```python
from build123d import *

# Parameters (mm, degrees)
AUFSATZ_LINEAR_AUSTRAGEN1_DEPTH      = 2.5
AUFSATZ_LINEAR_AUSTRAGEN1_DEPTH_BACK = 2.5
SKIZZE2_R                            = 1.5
SCHNITT_LINEAR_AUSTRAGEN1_DEPTH      = 3.5
SCHNITT_LINEAR_AUSTRAGEN1_DEPTH_BACK = 3.5
SCHNITT_LINEAR_AUSTRAGEN2_DEPTH      = 3.5
SCHNITT_LINEAR_AUSTRAGEN2_DEPTH_BACK = 3.5
SKIZZE7_W                            = 50
SKIZZE7_H                            = 20
AUFSATZ_LINEAR_AUSTRAGEN3_DEPTH      = 10
SCHNITT_LINEAR_AUSTRAGEN6_DEPTH      = 13.5
FASE1_SIZE                           = 2
SKETCH1_R                            = 3.175
CUT_EXTRUDE1_DEPTH                   = 10
SKETCH2_W                            = 15
SKETCH2_H                            = 3.5
BOSS_EXTRUDE1_DEPTH                  = 2.225
FILLET2_R                            = 5
FILLET1_R                            = 2


with BuildPart() as part:
    # Skizze1 → Aufsatz-Linear austragen1 (new body, two sides)
    with BuildSketch(Plane.XY) as aufsatz_linear_austragen1_sk:
        Polygon((-50, -20), (-50, 20), (50, 20), (50, -20), (25, -20), (25, -40), (-25, -40), (-25, -20), align=None)
    extrude(amount=AUFSATZ_LINEAR_AUSTRAGEN1_DEPTH)
    extrude(aufsatz_linear_austragen1_sk.sketch, amount=-AUFSATZ_LINEAR_AUSTRAGEN1_DEPTH_BACK)

    # Skizze2 → Schnitt-Linear austragen1 (cut, two sides)
    with BuildSketch(Plane.XY) as schnitt_linear_austragen1_sk:
        with Locations((-45, 15)):
            Circle(SKIZZE2_R)
        with Locations((-45, -15)):
            Circle(SKIZZE2_R)
        with Locations((45, -15)):
            Circle(SKIZZE2_R)
        with Locations((45, 15)):
            Circle(SKIZZE2_R)
    extrude(amount=SCHNITT_LINEAR_AUSTRAGEN1_DEPTH, mode=Mode.SUBTRACT)
    extrude(schnitt_linear_austragen1_sk.sketch, amount=-SCHNITT_LINEAR_AUSTRAGEN1_DEPTH_BACK, mode=Mode.SUBTRACT)

    # Skizze4 → Schnitt-Linear austragen2 (cut, two sides)
    with BuildSketch(Plane.XY) as schnitt_linear_austragen2_sk:
        with BuildLine():
            Line((-48, -8), (-48, 8))
            ThreePointArc((-48, 8), (-47.121320344, 10.121320344), (-45, 11))
            Line((-45, 11), (-40.5, 11))
            ThreePointArc((-40.5, 11), (-38.378679656, 10.121320344), (-37.5, 8))
            Line((-37.5, 8), (-37.5, -8))
            ThreePointArc((-37.5, -8), (-38.378679656, -10.121320344), (-40.5, -11))
            Line((-40.5, -11), (-45, -11))
            ThreePointArc((-45, -11), (-47.121320344, -10.121320344), (-48, -8))
        make_face()
        with BuildLine():
            Line((45, -11), (40.5, -11))
            ThreePointArc((40.5, -11), (38.378679656, -10.121320344), (37.5, -8))
            Line((37.5, -8), (37.5, 8))
            ThreePointArc((37.5, 8), (38.378679656, 10.121320344), (40.5, 11))
            Line((40.5, 11), (45, 11))
            ThreePointArc((45, 11), (47.121320344, 10.121320344), (48, 8))
            Line((48, 8), (48, -8))
            ThreePointArc((48, -8), (47.121320344, -10.121320344), (45, -11))
        make_face()
    extrude(amount=SCHNITT_LINEAR_AUSTRAGEN2_DEPTH, mode=Mode.SUBTRACT)
    extrude(schnitt_linear_austragen2_sk.sketch, amount=-SCHNITT_LINEAR_AUSTRAGEN2_DEPTH_BACK, mode=Mode.SUBTRACT)

    # Skizze7 → Aufsatz-Linear austragen3 (add)
    with BuildSketch(Plane(origin=(0, 0, -2.5), x_dir=(-1, 0, 0), z_dir=(0, 0, -1))):
        with Locations((0, -30)):
            Rectangle(SKIZZE7_W, SKIZZE7_H)
        Polygon((35, 20), (-35, 20), (-35, -20), (-25, -20), (25, -20), (35, -20), align=None)
    extrude(amount=AUFSATZ_LINEAR_AUSTRAGEN3_DEPTH)

    # Skizze8 → Schnitt-Linear austragen6 (cut)
    with BuildSketch(Plane.XY.offset(2.5)):
        with BuildLine():
            Line((30, 18), (-30, 18))
            ThreePointArc((-30, 18), (-32.121320344, 17.121320344), (-33, 15))
            Line((-33, 15), (-33, -15))
            ThreePointArc((-33, -15), (-32.121320344, -17.121320344), (-30, -18))
            Line((-30, -18), (30, -18))
            ThreePointArc((30, -18), (32.121320344, -17.121320344), (33, -15))
            Line((33, -15), (33, 15))
            ThreePointArc((33, 15), (32.121320344, 17.121320344), (30, 18))
        make_face()
        with BuildLine():
            Line((23, -18), (-23, -18))
            Line((-23, -18), (-23, -35))
            ThreePointArc((-23, -35), (-22.121320344, -37.121320344), (-20, -38))
            Line((-20, -38), (20, -38))
            ThreePointArc((20, -38), (22.121320344, -37.121320344), (23, -35))
            Line((23, -35), (23, -18))
        make_face()
    extrude(amount=-SCHNITT_LINEAR_AUSTRAGEN6_DEPTH, mode=Mode.SUBTRACT)

    # Fase1
    fase1_edges = [part.edges().sort_by_distance(p)[0] for p in [
        (-50, -20, 0),
        (-50, 20, 0),
        (50, 20, 0),
        (50, -20, 0),
        (25, -40, -5),
        (-25, -40, -5),
    ]]
    chamfer(fase1_edges, length=FASE1_SIZE)

    # Sketch1 → Cut-Extrude1 (cut)
    with BuildSketch(Plane(origin=(0, -40, 0), x_dir=(1, 0, 0), z_dir=(0, 1, 0))):
        with Locations((0, 4.25)):
            Circle(SKETCH1_R)
    extrude(amount=CUT_EXTRUDE1_DEPTH, mode=Mode.SUBTRACT)

    # Sketch2 → Boss-Extrude1 (add)
    with BuildSketch(Plane.XY.offset(-11)):
        with Locations((0, -36.25)):
            Rectangle(SKETCH2_W, SKETCH2_H)
    extrude(amount=BOSS_EXTRUDE1_DEPTH)

    # Fillet2
    fillet2_edges = [part.edges().sort_by_distance(p)[0] for p in [
        (-35, 0, -12.5),
        (35, 0, -12.5),
    ]]
    fillet(fillet2_edges, radius=FILLET2_R)

    # Fillet1
    fillet1_edges = [part.edges().sort_by_distance(p)[0] for p in [
        (-7.5, -36.25, -11),
        (7.5, -36.25, -11),
        (0, -34.5, -11),
    ]]
    fillet(fillet1_edges, radius=FILLET1_R)


solid = part.part
```
Geometry check sheet. Reference: the model listing, model coordinates, mm. A direction names the side the tool comes from. Coordinates: 2 decimals unless noted, no trailing zeros. Order: outer loops, then holes, each group sorted by start corner. A loop starts at its lowest first (then second) coordinate and runs counter-clockwise, first axis right, second up.
Item 1: Section check C-C (x = -19). Enter the section's corners in (y, z).
Item 2: Mould release check, pull along Z, two halves, no side actions. Record for faces 5 (the cylindrical face through (-8.1, -35.82, -10.43)), 6 (the cylindrical face through (-0.69, -39.01, -1.15)), 7 (the flat face through (35, 0, -5)): released by +Z, released by -Z, zero draft, split by the parting line, or undercut.
Item 3: Section check A-A (x = 0). Enter the section's corners in (y, z) (3 decimals).
Item 4: Scan lines: line 1 along Y through (x, z) = (-45, -1.05); line 2 along X through (y, z) = (15, 0.55); line 3 along X through (y, z) = (-26, -10.25). Record each from-to range of solid material in increasing order.
Item 5: Section check D-D (y = 9). Enter the section's corners in (x, z).
Item 6: Tool access check on faces 1 (the flat face through (-34, -20, -3)), 2 (the flat face through (24, -39, -5)), 3 (the cylindrical face through (-47.14, 10.1, 0.04)), 4 (the cylindrical face through (22.1, -37.14, -4.16)). Record the directions out of +Z, -Z, +X, -X, +Y, -Y that give a thin tool (end or side, any length) a straight path to the whole face; none if there is none.
Item 7: Depth check by flat-ended pin: pin 1 (1.3 mm diameter, centred on x = -42.5, z = 0.5, fed in from -Y); pin 2 (2.5 mm diameter, centred on x = -45, y = 15, fed in from -Z); pin 3 (6 mm diameter, centred on y = -26, z = -2.5, fed in from -X); pin 4 (7.5 mm diameter, centred on y = -33, z = -3, fed in from +X). Enter the tip coordinate at first touch or a pass-through.
Item 8: Section check B-B (y = 3). Enter the section's corners in (x, z).
Check sheet entries:
1. outline: (-40, -12.5) - (20, -12.5) - (20, 2.5) - (18, 2.5) - (18, -11) - (-38, -11) - (-38, 2.5) - (-40, 2.5) - close
2. face 5: released by +Z
2. face 6: undercut
2. face 7: zero draft
3. outline: (-40, -12.5) - (20, -12.5) - (20, 2.5) - (18, 2.5) - (18, -11) - (-32.5, -11) arc R2 cw to (-34.5, -9) - (-34.5, -8.775) - (-38, -8.775) - (-38, -7.425) - (-40, -7.425) - close; (-40, -1.075) - (-38, -1.075) - (-38, 2.5) - (-40, 2.5) - close
4. line 1: y = -20 to -16.5, -13.5 to -11, 11 to 13.5, 16.5 to 20
4. line 2: x = -50 to -46.5, -43.5 to -33, 33 to 43.5, 46.5 to 50
4. line 3: x = -25 to -23, 23 to 25
5. outline: (-50, -2.5) - (-47.83, -2.5) - (-47.83, 2.5) - (-50, 2.5) - close; (-37.67, -2.5) - (-35, -2.5) - (-35, -7.5) arc R5 ccw to (-30, -12.5) - (30, -12.5) arc R5 ccw to (35, -7.5) - (35, -2.5) - (37.67, -2.5) - (37.67, 2.5) - (33, 2.5) - (33, -11) - (-33, -11) - (-33, 2.5) - (-37.67, 2.5) - close; (47.83, -2.5) - (50, -2.5) - (50, 2.5) - (47.83, 2.5) - close
6. face 1: +Z, -Z, -X, -Y
6. face 2: +Z, -Z, +X, -Y
6. face 3: +Z, -Z
6. face 4: +Z
7. pin 1: stops at y = -20
7. pin 2: passes through
7. pin 3: stops at x = -25
7. pin 4: stops at x = 25
8. outline: (-50, -2.5) - (-48, -2.5) - (-48, 2.5) - (-50, 2.5) - close; (-37.5, -2.5) - (-35, -2.5) - (-35, -7.5) arc R5 ccw to (-30, -12.5) - (30, -12.5) arc R5 ccw to (35, -7.5) - (35, -2.5) - (37.5, -2.5) - (37.5, 2.5) - (33, 2.5) - (33, -11) - (-33, -11) - (-33, 2.5) - (-37.5, 2.5) - close; (48, -2.5) - (50, -2.5) - (50, 2.5) - (48, 2.5) - close
